from build123d import *

# Parameters (mm, degrees)
F0_W      = 18.542
F0_H      = 18.542
F1_DEPTH  = 8.89
F2_R      = 1.0287
F3_DEPTH  = 8.891
F5_D      = 3.175
F5_DEPTH  = 4.7752
F5_TIP    = 0.9538662327
F7_D      = 4.7752
F7_DEPTH  = 3.175
F7_TIP    = 1.434614814
F8_R      = 0.4064
F9_DEPTH  = 3.175
F10_R     = 1.4732
F11_DEPTH = 8.891
F12_W     = 18.542
F12_H     = 18.542
F12_R     = 5.715
F13_DEPTH = 2.54
F15_D     = 4.0386
F15_DEPTH = 5.55625
F15_TIP   = 1.213317848


with BuildPart() as f1:
    # F0 (on Top) → F1 (new body)
    with BuildSketch(Plane.XY):
        Rectangle(F0_W, F0_H)
    extrude(amount=F1_DEPTH)

    # F2 (on face) → F3 (cut, through all)
    with BuildSketch(Plane.XY.offset(8.89)):
        Circle(F2_R)
    extrude(amount=-F3_DEPTH, mode=Mode.SUBTRACT)

    # F5
    with Locations(Plane.XY.offset(8.89)):
        with Locations((0, 0)):
            Hole(F5_D / 2, depth=F5_DEPTH)
            with Locations((0, 0, -(F5_DEPTH + F5_TIP / 2))):  # 118° drill point
                Cone(0, F5_D / 2, F5_TIP, mode=Mode.SUBTRACT)

    # F7
    with Locations(Plane.XY.offset(8.89)):
        with Locations((0, 0)):
            Hole(F7_D / 2, depth=F7_DEPTH)
            with Locations((0, 0, -(F7_DEPTH + F7_TIP / 2))):  # 118° drill point
                Cone(0, F7_D / 2, F7_TIP, mode=Mode.SUBTRACT)

    # F8 (on face) → F9 (cut)
    with BuildSketch(Plane.XY.offset(8.89)):
        with Locations((-4.445, 0)):
            Circle(F8_R)
    extrude(amount=-F9_DEPTH, mode=Mode.SUBTRACT)

    # F10 (on face) → F11 (cut, through all)
    with BuildSketch(Plane.XY.offset(8.89)):
        with Locations((-6.985, 6.985)):
            Circle(F10_R)
        with Locations((-6.985, -6.985)):
            Circle(F10_R)
        with Locations((6.985, 6.985)):
            Circle(F10_R)
        with Locations((6.985, -6.985)):
            Circle(F10_R)
    extrude(amount=-F11_DEPTH, mode=Mode.SUBTRACT)

    # F12 (on face) → F13 (cut)
    with BuildSketch(Plane(origin=(0, 0, 0), x_dir=(1, 0, 0), z_dir=(0, 0, -1))):
        Rectangle(F12_W, F12_H)
        Circle(F12_R, mode=Mode.SUBTRACT)
    extrude(amount=-F13_DEPTH, mode=Mode.SUBTRACT)

    # F15
    with Locations(Plane(origin=(-9.271, 0, 0), x_dir=(0, -1, 0), z_dir=(-1, 0, 0))):
        with Locations((0, 5.715)):
            Hole(F15_D / 2, depth=F15_DEPTH)
            with Locations((0, 0, -(F15_DEPTH + F15_TIP / 2))):  # 118° drill point
                Cone(0, F15_D / 2, F15_TIP, mode=Mode.SUBTRACT)


solid = f1.part
The listing builds one solid part. Answer for the finished solid, in the listing's coordinates (mm). A direction names the side the tool comes from. Coordinates: 2 decimals unless noted, no trailing zeros. Loops run counter-clockwise (first coordinate to the right, second up) from the corner with the lowest first, then second, coordinate; pieces in that order, holes last.
1) Flat-ended cylindrical pins translate along their axes: pin 1 Ø2.5 at (x, y) = (-6.985, -6.985) entering from -Z; pin 2 Ø3.5 at (x, y) = (0, 0) entering from +Z; pin 3 Ø4 at (x, y) = (6.985, -6.985) entering from -Z. Find the tip coordinate at first contact, or state that the pin passes through.
2) Determine the mould class of faces 1 (the face through (-4.3, -4.3, 2.54)), 2 (the face through (0.5, -0.9, 1.9)), 3 (the face through (-2.712, -0.162, 5.404)) for opening direction X: pulls with the +X half, pulls with the -X half, needs draft (parallel to the pull), parting line crosses it, or undercut.
3) Find the intervals of material crossed by L1, parallel to X at y = 0, z = 8.3; L2, parallel to Y at x = 7.75, z = 8; L3, parallel to Y at x = 0, z = 7.95, in increasing order.
4) Find section C-C on y = 6.5. Write down the section's boundary in (x, z), then the cut area to 3 significant figures.
5) A tool of negligible diameter and unlimited length cuts with its end or side. For faces 4 (the face through (-6.454, -0.438, 3.744)), 5 (the face through (-7.177, 8.446, 5.759)), 6 (the face through (-4.057, 0.122, 8.3)), 7 (the face through (5.45, -1.72, 1.25)), 8 (the face through (0, 9.271, 6)), from which of +Z, -Z, +X, -X, +Y, -Y can it reach the whole face along a straight path? Write none if from no direction.
6) Find section A-A on x = 0. Write down the section's boundary in (y, z) (1 decimal).
7) Find section D-D on x = 6. Write down the section's boundary in (y, z).
8) Find section B-B on z = 3.25. Write down the section's boundary in (x, y) (3 decimals).
Values:
1. pin 1: passes through
1. pin 2: stops at z = 5.33
1. pin 3: stops at z = 2.54
2. face 1: needs draft
2. face 2: undercut
2. face 3: pulls with the -X half
3. L1: x = -9.27 to -4.85, -4.04 to -2.39, 2.39 to 9.27
3. L2: y = -9.27 to -8.24, -5.73 to 5.73, 8.24 to 9.27
3. L3: y = -9.27 to -2.39, 2.39 to 9.27
4. outline: (-9.27, 2.54) - (-8.38, 2.54) - (-8.38, 8.89) - (-9.27, 8.89) - close; (-5.59, 2.54) - (5.59, 2.54) - (5.59, 8.89) - (-5.59, 8.89) - close; (8.38, 2.54) - (9.27, 2.54) - (9.27, 8.89) - (8.38, 8.89) - close
4. area: 82.4 mm2
5. face 4: -X
5. face 5: +Z, -Z
5. face 6: +Z
5. face 7: -Z
5. face 8: +Z, -Z, +X, -X, +Y
6. outline: (-9.3, 2.5) - (-5.7, 2.5) - (-5.7, 0) - (-1, 0) - (-1, 3.8) - (-1.6, 4.1) - (-1.6, 5.2) - (-2.4, 5.7) - (-2.4, 8.9) - (-9.3, 8.9) - close; (1, 0) - (5.7, 0) - (5.7, 2.5) - (9.3, 2.5) - (9.3, 8.9) - (2.4, 8.9) - (2.4, 5.7) - (1.6, 5.2) - (1.6, 4.1) - (1, 3.8) - close
7. outline: (-9.27, 2.54) - (-8.08, 2.54) - (-8.08, 8.89) - (-9.27, 8.89) - close; (-5.89, 2.54) - (5.89, 2.54) - (5.89, 8.89) - (-5.89, 8.89) - close; (8.08, 2.54) - (9.27, 2.54) - (9.27, 8.89) - (8.08, 8.89) - close
8. outline: (-9.271, -9.271) - (9.271, -9.271) - (9.271, 9.271) - (-9.271, 9.271) - close; hole circle Ø2.946 at (-6.985, -6.985); hole circle Ø2.946 at (-6.985, 6.985); hole circle Ø2.057 at (0, 0); hole circle Ø2.946 at (6.985, -6.985); hole circle Ø2.946 at (6.985, 6.985)
